from build123d import *

# Parameters (mm, degrees)
SKETCH_1_W          = 20
SKETCH_1_H          = 20
SKETCH_1_W_2        = 18
SKETCH_1_H_2        = 18
EXTRUDE_1_DEPTH     = 500
CUT_EXTRUDE_1_REACH = 502.5
SKETCH_2_R          = 1.6


with BuildPart() as part:
    # 草图1 → 凸台-拉伸1 (new body)
    with BuildSketch(Plane.XY):
        Rectangle(SKETCH_1_W, SKETCH_1_H)
        Rectangle(SKETCH_1_W_2, SKETCH_1_H_2, mode=Mode.SUBTRACT)
    extrude(amount=EXTRUDE_1_DEPTH)

    # 切除-拉伸1: up to this face of the body (flat: up to its plane)
    cut_extrude_1_end = Plane(part.part.faces().sort_by_distance((10, 0, 250))[0])
    # 草图2 → 切除-拉伸1 (cut, up to the picked face)
    with BuildSketch(Plane.ZY.offset(10), mode=Mode.PRIVATE) as cut_extrude_1_sk1:
        with Locations((15, -4)):
            Circle(SKETCH_2_R)
    cut_extrude_1_tool1 = split(extrude(cut_extrude_1_sk1.sketch, amount=-CUT_EXTRUDE_1_REACH, mode=Mode.PRIVATE), bisect_by=cut_extrude_1_end, keep=Keep.BOTH, mode=Mode.PRIVATE)
    # 草图2 → 切除-拉伸1 (cut, up to the picked face)
    with BuildSketch(Plane.ZY.offset(10), mode=Mode.PRIVATE) as cut_extrude_1_sk2:
        with Locations((15, 4)):
            Circle(SKETCH_2_R)
    cut_extrude_1_tool2 = split(extrude(cut_extrude_1_sk2.sketch, amount=-CUT_EXTRUDE_1_REACH, mode=Mode.PRIVATE), bisect_by=cut_extrude_1_end, keep=Keep.BOTH, mode=Mode.PRIVATE)
    # 草图2 → 切除-拉伸1 (cut, up to the picked face)
    with BuildSketch(Plane.ZY.offset(10), mode=Mode.PRIVATE) as cut_extrude_1_sk3:
        with Locations((8.07179677, 0)):
            Circle(SKETCH_2_R)
    cut_extrude_1_tool3 = split(extrude(cut_extrude_1_sk3.sketch, amount=-CUT_EXTRUDE_1_REACH, mode=Mode.PRIVATE), bisect_by=cut_extrude_1_end, keep=Keep.BOTH, mode=Mode.PRIVATE)
    # 草图2 → 切除-拉伸1 (cut, up to the picked face)
    with BuildSketch(Plane.ZY.offset(10), mode=Mode.PRIVATE) as cut_extrude_1_sk4:
        with Locations((21.92820323, 0)):
            Circle(SKETCH_2_R)
    cut_extrude_1_tool4 = split(extrude(cut_extrude_1_sk4.sketch, amount=-CUT_EXTRUDE_1_REACH, mode=Mode.PRIVATE), bisect_by=cut_extrude_1_end, keep=Keep.BOTH, mode=Mode.PRIVATE)
    # 草图2 → 切除-拉伸1 (cut, up to the picked face)
    with BuildSketch(Plane.ZY.offset(10), mode=Mode.PRIVATE) as cut_extrude_1_sk5:
        with Locations((478.07179677, 0)):
            Circle(SKETCH_2_R)
    cut_extrude_1_tool5 = split(extrude(cut_extrude_1_sk5.sketch, amount=-CUT_EXTRUDE_1_REACH, mode=Mode.PRIVATE), bisect_by=cut_extrude_1_end, keep=Keep.BOTH, mode=Mode.PRIVATE)
    # 草图2 → 切除-拉伸1 (cut, up to the picked face)
    with BuildSketch(Plane.ZY.offset(10), mode=Mode.PRIVATE) as cut_extrude_1_sk6:
        with Locations((485, 4)):
            Circle(SKETCH_2_R)
    cut_extrude_1_tool6 = split(extrude(cut_extrude_1_sk6.sketch, amount=-CUT_EXTRUDE_1_REACH, mode=Mode.PRIVATE), bisect_by=cut_extrude_1_end, keep=Keep.BOTH, mode=Mode.PRIVATE)
    # 草图2 → 切除-拉伸1 (cut, up to the picked face)
    with BuildSketch(Plane.ZY.offset(10), mode=Mode.PRIVATE) as cut_extrude_1_sk7:
        with Locations((485, -4)):
            Circle(SKETCH_2_R)
    cut_extrude_1_tool7 = split(extrude(cut_extrude_1_sk7.sketch, amount=-CUT_EXTRUDE_1_REACH, mode=Mode.PRIVATE), bisect_by=cut_extrude_1_end, keep=Keep.BOTH, mode=Mode.PRIVATE)
    # 草图2 → 切除-拉伸1 (cut, up to the picked face)
    with BuildSketch(Plane.ZY.offset(10), mode=Mode.PRIVATE) as cut_extrude_1_sk8:
        with Locations((491.92820323, 0)):
            Circle(SKETCH_2_R)
    cut_extrude_1_tool8 = split(extrude(cut_extrude_1_sk8.sketch, amount=-CUT_EXTRUDE_1_REACH, mode=Mode.PRIVATE), bisect_by=cut_extrude_1_end, keep=Keep.BOTH, mode=Mode.PRIVATE)
    add(cut_extrude_1_tool1.solids().sort_by(Axis((-10, -4, 15), (1, 0, 0)))[0], mode=Mode.SUBTRACT)
    add(cut_extrude_1_tool2.solids().sort_by(Axis((-10, 4, 15), (1, 0, 0)))[0], mode=Mode.SUBTRACT)
    add(cut_extrude_1_tool3.solids().sort_by(Axis((-10, 0, 8.071797), (1, 0, 0)))[0], mode=Mode.SUBTRACT)
    add(cut_extrude_1_tool4.solids().sort_by(Axis((-10, 0, 21.928203), (1, 0, 0)))[0], mode=Mode.SUBTRACT)
    add(cut_extrude_1_tool5.solids().sort_by(Axis((-10, 0, 478.071797), (1, 0, 0)))[0], mode=Mode.SUBTRACT)
    add(cut_extrude_1_tool6.solids().sort_by(Axis((-10, 4, 485), (1, 0, 0)))[0], mode=Mode.SUBTRACT)
    add(cut_extrude_1_tool7.solids().sort_by(Axis((-10, -4, 485), (1, 0, 0)))[0], mode=Mode.SUBTRACT)
    add(cut_extrude_1_tool8.solids().sort_by(Axis((-10, 0, 491.928203), (1, 0, 0)))[0], mode=Mode.SUBTRACT)


solid = part.part
Here's how the part is built. I have some questions about the finished solid (model axes, mm). A direction names the side the tool comes from. Round coordinates to 2 decimals unless told otherwise and drop trailing zeros. Loops run counter-clockwise (first coordinate to the right, second up) from the corner with the lowest first, then second, coordinate; pieces in that order, holes last. Notation, with made-up numbers: (40.25, 59.5) - (52.25, 59.5) arc R24 ccw to (52.25, 77.5) - close; hole circle Ø8 at (11.5, 42.25). An arc over 180 degrees is marked (long way). One line per question, with ' | ' between items. Start each with the question number.
Q1. Please list where these lines run through material, in increasing order: line 1 (Y direction, x = -9.25, z = 15); line 2 (X direction, y = 0.5, z = 327.5). Write a range as [from, to].
Q2. I want a section at B-B (z = 302). Write out the boundary of the cut face in (x, y), then the cut area to 3 significant figures.
Q3. For faces 1 (the flat face through (0, -9, 246)), 2 (the flat face through (-0.8, -9.6, 0)), which set-ups out of +Z, -Z, +X, -X, +Y, -Y let a thin tool reach every point of the face, with its end or its side?
Q4. I want a section at A-A (x = -6). Write out the boundary of the cut face in (y, z), then the cut area to 3 significant figures.
Q5. We'd pull the mould along Y, two halves only. Please class faces 3 (the flat face through (9, 0, 246)), 4 (the flat face through (-10, 0, 246)), 5 (the flat face through (0, -10, 246)), 6 (the flat face through (0, 10, 246)): +Y half, -Y half, draft (parallel to the pull), parting line (faces both ways), or undercut.
Response values:
1) line 1: y = [-10, -5.6], [-2.4, 2.4], [5.6, 10] | line 2: x = [-10, -9], [9, 10]
2) outline: (-10, -10) - (10, -10) - (10, 10) - (-10, 10) - close; hole (-9, -9) - (9, -9) - (9, 9) - (-9, 9) - close | area: 76.0 mm²
3) face 1: +Z, -Z | face 2: -Z, +X, -X, +Y, -Y
4) outline: (-10, 0) - (-9, 0) - (-9, 500) - (-10, 500) - close; (9, 0) - (10, 0) - (10, 500) - (9, 500) - close | area: 1,000 mm²
5) face 3: undercut | face 4: draft | face 5: -Y half | face 6: +Y half
